Can you work these out from the model? Positions are in its coordinate system, mm. A direction names the side the tool comes from. Coordinates: 2 decimals unless noted, no trailing zeros. Order: outer loops, then holes, each group sorted by start corner. A loop starts at its lowest first (then second) coordinate and runs counter-clockwise, first axis right, second up. Notation, with made-up numbers: M 24.5,60.5 L 50.5,60.5 A28 ccw 50.5,84.5 Z; hole C 25,61.5 d10. An arc over 180 degrees is marked long. Answer as a JSON object with one key per item and string values.
Autodesk Inventor part; units mm, degrees
ref_plane "YZ Plane" through (0, 0, 0) normal (1, 0, 0) x (0, 1, 0)
ref_plane "XZ Plane" through (0, 0, 0) normal (0, 1, 0) x (-1, 0, 0)
ref_plane "XY Plane" through (0, 0, 0) normal (0, 0, 1) x (1, 0, 0)
sketch "Sketch1" plane through (0, 0, 0) normal (0, 1, 0) x (-1, 0, 0)
  circle A0 centre (0, 0) radius 8.15
  circle A1 centre (0, 0) radius 10
  dimension "d0" = 16.3
  dimension "d1" = 20
extrude "Extrusion1" add sketch "Sketch1" along normal blind 5
sketch "Sketch2" plane through (0, 5, 0) normal (0, 1, 0) x (1, 0, 0)
  circle A0 centre (0, 0) radius 10
  circle A1 centre (0, 0) radius 8.15
  circle A2 centre (0, 0) radius 17.5
  dimension "d4" = 35
extrude "Extrusion2" add sketch "Sketch2" along normal blind 4 contours A0 | A2
chamfer "Chamfer1" distance 0.5 angle 45 2 edges at (10, 0, 0) (-8.15, 9, 0)
properties part number "Ydre_bøsning_stempel_stang"
Item 1: I want a section at C-C, the plane z = 12. Write out the boundary of the cut face in (x, y).
Answers follow:
{"outline": "M -12.74,5 L 12.74,5 L 12.74,9 L -12.74,9 Z"}
Item 2: I'm going to push flat-ended pins straight in: pin 1 (6 mm diameter, centred on x = 11, z = -13.5, fed in from -Y); pin 2 (10 mm diameter, centred on x = 0, z = 0, fed in from -Y); pin 3 (1 mm diameter, centred on y = 3, z = 1, fed in from +X); pin 4 (3 mm diameter, centred on y = 7, z = -10, fed in from -X). Where does each tip first touch, or does it pass through?
Answers follow:
{"pin 1": "stops at y = 5", "pin 2": "passes through", "pin 3": "stops at x = 9.99", "pin 4": "stops at x = -15.3"}
Item 3: Which directions (+Z, -Z, +X, -X, +Y, -Y) give clear straight access to the entire face, cutting with the end or side of a thin tool? Please do faces 1 (the flat face through (8, 5, 8)), 2 (the flat face through (-3, 0, 8)).
Answers follow:
{"face 1": "-Y", "face 2": "+Z, -Z, +X, -X, -Y"}
Item 4: If we mould it in two halves opening along X, with no side actions, what happens to faces 3 (the cylindrical face through (-13.887, 6.972, -10.648)), 4 (the cylindrical face through (0.537, 5.135, 8.132)), 5 (the flat face through (-8, 9, 4))? For each: pulls with the +X half, pulls with the -X half, needs draft (parallel to the pull), parting line crosses it, or undercut.
Answers follow:
{"face 3": "parting line crosses it", "face 4": "undercut", "face 5": "needs draft"}
Item 5: I want a section at D-D, the plane x = 13. Write out the boundary of the cut face in (y, z).
Answers follow:
{"outline": "M 5,-11.72 L 9,-11.72 L 9,11.72 L 5,11.72 Z"}
Item 6: I want a section at B-B, the plane y = 3.5. Write out the boundary of the cut face in (x, z).
Answers follow:
{"outline": "C 0,0 d20; hole C 0,0 d16.3"}
Item 7: Please list where these lines run through material, in increasing order: line 1 (Z direction, x = 0, y = 4.25); line 2 (X direction, y = 6, z = 0); line 3 (X direction, y = 8.5, z = -4).
Answers follow:
{"line 1": "z = -10 to -8.15, 8.15 to 10", "line 2": "x = -17.5 to -8.15, 8.15 to 17.5", "line 3": "x = -17.04 to -7.1, 7.1 to 17.04"}
